Verification items for this drawing (mm, ordinates from the low corner). A direction names the side the tool comes from. Give positions to 0.01 mm unless a question says otherwise; leave off trailing zeros. Write each loop counter-clockwise with the first axis right and the second up, starting at its lowest first coordinate (ties: lowest second). Pieces come first, ordered by that corner, then holes. Notation, with made-up numbers: (-14, 39) -> (17, 39) arc R18 ccw to (17, 64) -> close; hole circle Ø7 at (23.5, 9). An arc over 180 degrees is marked (long way). Use one line per item in the form item = value. Start each with the question number.
(1) Set-up check for the marked faces 4, 5 and 6: record each of +Z, -Z, +X, -X, +Y, -Y from which the full face is reachable in a straight line by a thin tool's end or side.
(2) Scan lines: L1, parallel to Z at x = 5.75, y = 1.5; L2, parallel to Y at x = 55.5, z = 2.5; L3, parallel to X at y = 1.5, z = 21.5 (1 decimal). Record each from-to range of solid material in increasing order.
(3) Depth check by flat-ended pin: pin 1 Ø5.5 at (x, z) = (60.61, 16.5) entering from -Y; pin 2 Ø10 at (x, z) = (45, 22) entering from +Y; pin 3 Ø3.5 at (x, z) = (7, 9) entering from +Y; pin 4 Ø8 at (x, z) = (23.5, 21.5) entering from -Y. Enter the tip coordinate at first touch or a pass-through.
(4) Release check for a two-part mould opening along Z. For the marked faces 1, 2 and 3 record: pulls with the +Z half, pulls with the -Z half, needs draft (parallel to the pull), parting line crosses it, or undercut.
(5) Section check C-C, the plane z = 16.5. Record the cut outline in (x, y).
(6) Section check B-B, the plane y = 3.75. Record the cut outline in (x, z), plus the area to 3 significant figures.
(7) Section check A-A, the plane x = 5.75. Record the cut outline in (y, z), plus the area to 3 significant figures.
(8) Section check D-D, the plane y = 12. Record the cut outline in (x, z).
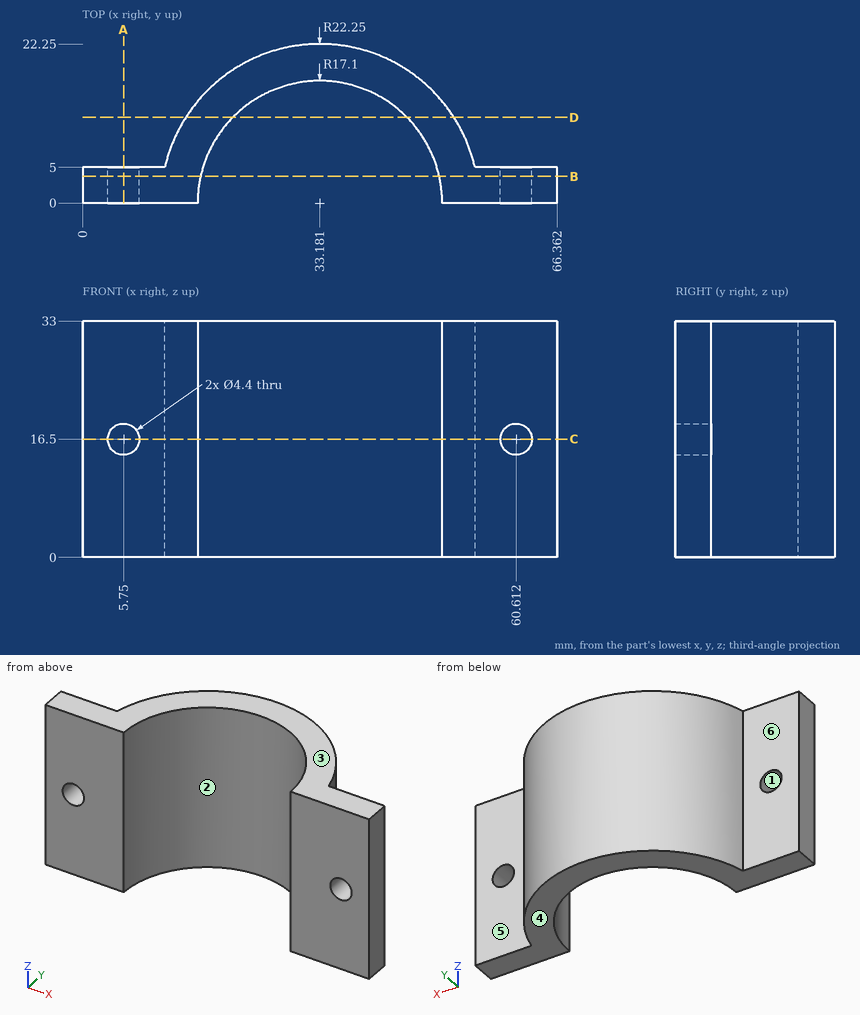
Completed:
q1.face_4 = -Z, +X, -X, +Y, -Y
q1.face_5 = +Z, -Z, +X, +Y
q1.face_6 = +Z, -Z, -X, +Y
q2.L1 = 0 to 14.3, 18.7 to 33
q2.L2 = 0 to 5
q2.L3 = 0 to 16.1, 50.2 to 66.4
q3.pin_1 = 0
q3.pin_2 = 21.18
q3.pin_3 = 5
q3.pin_4 = 10.26
q4.face_1 = undercut
q4.face_2 = needs draft
q4.face_3 = pulls with the +Z half
q5.outline = (0, 0) -> (3.55, 0) -> (3.55, 5) -> (0, 5) -> close; (7.95, 0) -> (16.08, 0) arc R17.1 cw to (50.28, 0) -> (58.41, 0) -> (58.41, 5) -> (54.86, 5) arc R22.25 ccw to (11.5, 5) -> (7.95, 5) -> close; (62.81, 0) -> (66.36, 0) -> (66.36, 5) -> (62.81, 5) -> close
q6.outline = (0, 0) -> (16.5, 0) -> (16.5, 33) -> (0, 33) -> close; (49.86, 0) -> (66.36, 0) -> (66.36, 33) -> (49.86, 33) -> close; hole circle Ø4.4 at (5.75, 16.5); hole circle Ø4.4 at (60.61, 16.5)
q6.area = 1,060 mm²
q7.outline = (0, 0) -> (5, 0) -> (5, 14.3) -> (0, 14.3) -> close; (0, 18.7) -> (5, 18.7) -> (5, 33) -> (0, 33) -> close
q7.area = 143 mm²
q8.outline = (14.44, 0) -> (21, 0) -> (21, 33) -> (14.44, 33) -> close; (45.36, 0) -> (51.92, 0) -> (51.92, 33) -> (45.36, 33) -> close
